Build history of the part. All positions in model axes, mm. Face numbers are marked on the shaded views. A direction names the side the tool comes from. Round coordinates to 2 decimals unless told otherwise and drop trailing zeros. Write each loop counter-clockwise with the first axis right and the second up, starting at its lowest first coordinate (ties: lowest second). Pieces come first, ordered by that corner, then holes.
Solid Edge part; units mm, degrees
sketch "Sketch1" plane through (0, 0, 0) normal (0, -1, 0) x (1, 0, 0)
  line L0 (60, 0) -> (60, 110)
  line L1 (60, 110) -> (0, 110)
  line L2 (0, 110) -> (0, 0)
  line L3 (0, 0) -> (60, 0)
  circle A0 centre (30, 93.6) radius 5.1
  circle A1 centre (30, 36.4) radius 5.1
  circle A2 centre (30, 65) radius 20.5
extrude "Protrusion1" add sketch "Sketch1" along normal blind 10
sketch "Sketch2" plane through (0, 0, 0) normal (0, -1, 0) x (1, 0, 0)
  line L0 (0, 20) -> (60, 20)
  line L1 (60, 20) -> (60, 0)
  line L2 (60, 0) -> (0, 0)
  line L3 (0, 0) -> (0, 20)
extrude "övre_fäste_protrusion" add sketch "Sketch2" along normal blind 50
hole "Hole_5" at (10, -40, 0) direction (0, 0, 1) diameter 6.647 depth 15
hole "Hole1" at (50, -40, 0) direction (0, 0, 1) diameter 6.647 depth 15
hole "Hole2" at (10, -10, 0) direction (0, 0, 1) diameter 6.647 depth 15
hole "Hole3" at (50, -10, 0) direction (0, 0, 1) diameter 6.647 depth 15
fillet "Round_1" radius 5 10 edges at (0, -5, 110) (60, -5, 110) (30, -10, 20) (30, -50, 20) (0, -30, 20) (60, -30, 20) (60, -10, 65) (0, -10, 65) (30, -10, 110) (30, 0, 110)
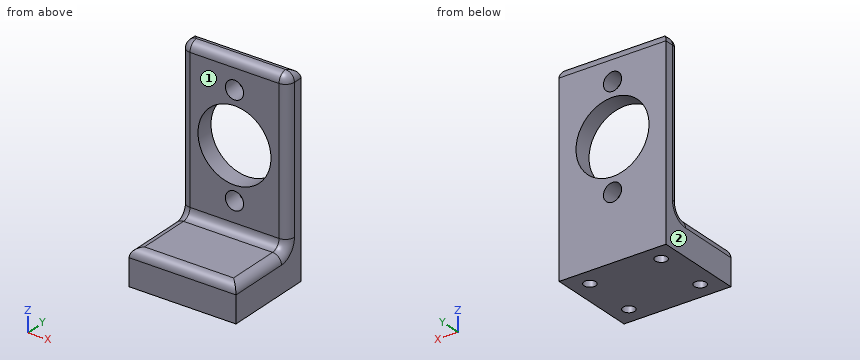
1) Pin check, flat tips, straight feed: pin 1 Ø2 at (x, y) = (10, -40) entering from -Z; pin 2 Ø12 at (x, y) = (52, -21) entering from +Z; pin 3 Ø2 at (y, z) = (-6.5, 66.5) entering from +X (3 decimals). Stop position of each tip, or through.
Results:
pin 1: stops at z = 15
pin 2: stops at z = 20
pin 3: stops at x = 59.975
2) Wall check: L1, parallel to Z at x = 30, y = -5.25; L2, parallel to X at y = -40, z = 7; L3, parallel to Y at x = 50, z = 3. Give the ranges that are in metal, low to high.
Results:
L1: z = 0 to 31.3, 41.5 to 44.5, 85.5 to 88.5, 98.7 to 109.99
L2: x = 0 to 6.68, 13.32 to 46.68, 53.32 to 60
L3: y = -50 to -43.32, -36.68 to -13.32, -6.68 to 0
3) Slice it at C-C (z = 65). Write the cut outline in (x, y).
Results:
outline: (0, -5) arc R5 ccw to (5, -10) - (9.5, -10) - (9.5, 0) - (0, 0) - close; (50.5, -10) - (55, -10) arc R5 ccw to (60, -5) - (60, 0) - (50.5, 0) - close
4) Which spindle directions (+Z, -Z, +X, -X, +Y, -Y) get a long thin tool onto all of the face, cutting with end or side? Do the marked faces 1 and 2. Say none if no direction does.
Results:
face 1: +Z, +X, -X, -Y
face 2: +Z, -Z, -X, +Y, -Y
5) Slice it at B-B (x = 30). Count the separate pieces of the cut face and the enclosed holes in it, plus the area to 3 significant figures.
Results:
separate pieces: 4
enclosed holes: 0
area: 1,280 mm2
6) Slice it at A-A (z = 93.6). Write the cut outline in (x, y), plus the area to 3 significant figures.
Results:
outline: (0, -5) arc R5 ccw to (5, -10) - (24.9, -10) - (24.9, 0) - (0, 0) - close; (35.1, -10) - (55, -10) arc R5 ccw to (60, -5) - (60, 0) - (35.1, 0) - close
area: 487 mm2
